Here's how the part is built. I have some questions about the finished solid (model axes, mm). A direction names the side the tool comes from. Give positions to 0.01 mm unless a question says otherwise; leave off trailing zeros. Write each loop counter-clockwise with the first axis right and the second up, starting at its lowest first coordinate (ties: lowest second). Pieces come first, ordered by that corner, then holes. Notation, with made-up numbers: M 12,8 L 57,8 A23 ccw 57,45 Z; hole C 68,86 d9. An arc over 180 degrees is marked long. Use one line per item in the form item = value. Start each with the question number.
Autodesk Inventor part; units mm, degrees
ref_plane "YZ Plane" through (0, 0, 0) normal (1, 0, 0) x (0, 1, 0)
ref_plane "XZ Plane" through (0, 0, 0) normal (0, 1, 0) x (-1, 0, 0)
ref_plane "XY Plane" through (0, 0, 0) normal (0, 0, 1) x (1, 0, 0)
sketch "스케치1" plane through (0, 0, 0) normal (0, 0, 1) x (1, 0, 0)
  circle A0 centre (0, 0) radius 45
  dimension "d0" = 90
extrude "돌출1" add sketch "스케치1" along normal blind 3
sketch "스케치2" plane through (0, 0, 3) normal (0, 0, 1) x (1, 0, 0)
  circle A0 centre (0, 0) radius 45
  circle A1 centre (0, 0) radius 37.5
  dimension "d3" = 75
extrude "돌출2" add sketch "스케치2" along normal blind 3 contours A1
sketch "스케치3" plane through (0, 0, 6) normal (0, 0, 1) x (1, 0, 0)
  circle A0 centre (0, 0) radius 37.5
  circle A1 centre (0, 0) radius 45
  dimension "d6" = 90
extrude "돌출3" add sketch "스케치3" along normal blind 5 contours A0 | A1
sketch "스케치4" plane through (0, 0, 11) normal (0, 0, 1) x (1, 0, 0)
  circle A0 centre (0, 0) radius 45
  circle A1 centre (0, 0) radius 3.2
  line L0 (-2.5, -1.9975) -> (-2.5, 1.9975)
  circle A2 centre (0, 0) radius 35
  line L1 (4, 0) -> (-4, 0)
  line L2 (-4, 0) -> (-4, -35)
  line L3 (-4, -35) -> (4, -35)
  line L4 (4, -35) -> (4, 0)
  line L5 (32.3109, -14.0359) -> (2, 3.4641)
  line L6 (-2, -3.4641) -> (28.3109, -20.9641)
  line L7 (28.3109, -20.9641) -> (32.3109, -14.0359)
  line L8 (2, 3.4641) -> (-2, -3.4641)
  line L9 (28.3109, 20.9641) -> (-2, 3.4641)
  line L10 (2, -3.4641) -> (32.3109, 14.0359)
  line L11 (32.3109, 14.0359) -> (28.3109, 20.9641)
  line L12 (-2, 3.4641) -> (2, -3.4641)
  line L13 (-4, 35) -> (-4, 0)
  line L14 (4, 0) -> (4, 35)
  line L15 (4, 35) -> (-4, 35)
  line L16 (-4, 0) -> (4, 0)
  line L17 (-32.3109, 14.0359) -> (-2, -3.4641)
  line L18 (2, 3.4641) -> (-28.3109, 20.9641)
  line L19 (-28.3109, 20.9641) -> (-32.3109, 14.0359)
  line L20 (-2, -3.4641) -> (2, 3.4641)
  line L21 (-28.3109, -20.9641) -> (2, -3.4641)
  line L22 (-2, 3.4641) -> (-32.3109, -14.0359)
  line L23 (-32.3109, -14.0359) -> (-28.3109, -20.9641)
  line L24 (2, -3.4641) -> (-2, 3.4641)
  point P0 (32.1123, 13.9212)
  point P1 (8, 0)
  point P2 (32.1123, -13.9212)
  point P3 (4, 34.7707)
  point P4 (4, 6.9282)
  point P5 (28.1123, 20.8494)
  point P6 (-28.1123, 20.8494)
  point P7 (-4, 6.9282)
  point P8 (-4, 34.7707)
  point P9 (-32.1123, -13.9212)
  point P10 (-8, 0)
  point P11 (-32.1123, 13.9212)
  point P12 (-4, -6.9282)
  point P13 (-28.1123, -20.8494)
  point P14 (-4, -34.7707)
  point P15 (28.1123, -20.8494)
  point P16 (4, -6.9282)
  point P17 (4, -34.7707)
  point P18 (0, 0)
  point P19 (0, 0)
  point P20 (0, 0)
  point P21 (0, 0)
  point P22 (0, 0)
  point P23 (0, 0)
  dimension "d10" = 6.4
  dimension "d11" = 2.5
  dimension "d14" = 70
  dimension "d15" = 8
  dimension "d16" = 35
  dimension "d19" = 360
extrude "돌출4" cut sketch "스케치4" against normal through all contours L1 L8 A1 | A1 L12 L1 | L8 L12 A1 | A1 L8 L12 | L8 A1 L0 L1 | L1 L0 A1 L12 | L6 A2 L4 | L10 A2 L5 | L14 A2 L9 | L18 A2 L13 | L2 A2 L21 | L22 A2 L17
fillet "모깎기2" radius 1 36 edges at (-20.0561, -6.9606, 11) (-16.0561, -13.8888, 11) (-35, 0, 11) (-20.0561, 6.9606, 11) (-16.0561, 13.8888, 11) (-17.5, 30.3109, 11) (-4, 20.8494, 11) (4, 20.8494, 11) (17.5, 30.3109, 11) (16.0561, 13.8888, 11) (20.0561, 6.9606, 11) (20.0561, 6.9606, 0) (35, 0, 11) (4, 20.8494, 0) (17.5, 30.3109, 0) (20.0561, -6.9606, 11) (16.0561, -13.8888, 11) (4, -20.8494, 11) (4, -20.8494, 0) (16.0561, -13.8888, 0) (-4, -20.8494, 11) (-16.0561, -13.8888, 0) (-20.0561, 6.9606, 0) (-17.5, 30.3109, 0) (-35, 0, 0) (-17.5, -30.3109, 0) (-17.5, -30.3109, 11) (-4, -20.8494, 0) (17.5, -30.3109, 11) (17.5, -30.3109, 0) (35, 0, 0) (20.0561, -6.9606, 0) (-4, 20.8494, 0) (-16.0561, 13.8888, 0) (16.0561, 13.8888, 0) (-20.0561, -6.9606, 0)
chamfer "모따기1" distance 3 distance2 1 1 edges at (-45, 0, 3) measured on face at (42.1722, 3.1187, 3)
properties part number "_3D 인쇄"
1) On a 3-axis mill with a long thin cutter (end or side, diameter ignored), from which of +Z, -Z, +X, -X, +Y, -Y can I reach the whole of each face in a straight line? I mean faces 4 (the face through (16.121, -13.579, 10.715)), 5 (the face through (19.456, -6.943, 0.301)), 6 (the face through (-17.67, -30.21, 5.56)). Say none if no direction works.
2) Suppose I cut it at A-A, the plane x = 0. List the corners of the cut face in (y, z) for me.
3) Please list where these lines run through material, in increasing order: line 1 (Y direction, x = 0, z = 4); line 2 (X direction, y = 15, z = 10.75); line 3 (X direction, y = 29, z = 7.75).
4) Suppose I cut it at C-C, the plane y = -27.5. State how many separate pieces and enclosed holes the cut face has, and give its area (3 significant figures).
5) Will these pins go through, and if not, where does the flat tip stop? P1, Ø3, axis at x = -15.5, z = 1.5, coming from the -Y side; P2, Ø4.5, axis at y = -17.5, z = 5, coming from the -X side; P3, Ø4, axis at x = 14, z = 6, coming from the +Y side.
6) Suppose I cut it at B-B, the plane z = 7.5. List the corners of the cut face in (x, y) for me.
7) Thinking about a two-plate mould opening in Y: for faces 1 (the face through (-17.33, 30.41, 5.56)), 2 (the face through (20.765, 39.923, 8.465)), 3 (the face through (-15.8, 34.4, 3)), which applies, released by +Y, released by -Y, zero draft, split by the parting line, or undercut?
Checks:
q1.face_4 = +Z
q1.face_5 = -Z
q1.face_6 = +Z, -Z
q2.outline = M -45,0 L -3.2,0 L -3.2,11 L -45,11 L -45,6 L -37.5,6 L -37.5,3 L -42,3 L -45,2 Z; M 3.2,0 L 45,0 L 45,2 L 42,3 L 37.5,3 L 37.5,6 L 45,6 L 45,11 L 3.2,11 Z
q3.line_1 = -37.5 to -3.2, 3.2 to 37.5
q3.line_2 = -42.43 to -18.66, -3.66 to 3.66, 18.66 to 42.43
q3.line_3 = -34.41 to -19.6, -4 to 4, 19.6 to 34.41
q4.separate_pieces = 3
q4.enclosed_holes = 0
q4.area = 328 mm^2
q5.P1 = -42.77
q5.P2 = -42.25
q5.P3 = 43.37
q6.outline = C 0,0 d90; hole M -32.11,-13.92 L -8,0 L -32.11,13.92 A35 ccw Z; hole M -28.11,-20.85 A35 ccw -4,-34.77 L -4,-6.93 Z; hole M -28.11,20.85 L -4,6.93 L -4,34.77 A35 ccw Z; hole M -2.5,-2 A3.2 ccw long -2.5,2 Z; hole M 4,-34.77 A35 ccw 28.11,-20.85 L 4,-6.93 Z; hole M 4,6.93 L 28.11,20.85 A35 ccw 4,34.77 Z; hole M 8,0 L 32.11,-13.92 A35 ccw 32.11,13.92 Z
q7.face_1 = undercut
q7.face_2 = split by the parting line
q7.face_3 = zero draft
